Geometry: final body of the model. Coordinates: model frame, mm. Face numbers are marked on the shaded views. A direction names the side the tool comes from. Coordinates: 2 decimals unless noted, no trailing zeros. Loops run counter-clockwise (first coordinate to the right, second up) from the corner with the lowest first, then second, coordinate; pieces in that order, holes last. Notation, with made-up numbers: (-17, 47.25) - (29, 47.25) arc R26 ccw to (29, 75.25) - close; hole circle Ø8 at (27.5, -11.5). An arc over 180 degrees is marked (long way). Write each question's results on one line, items separated by ' | '. Start each with the question number.
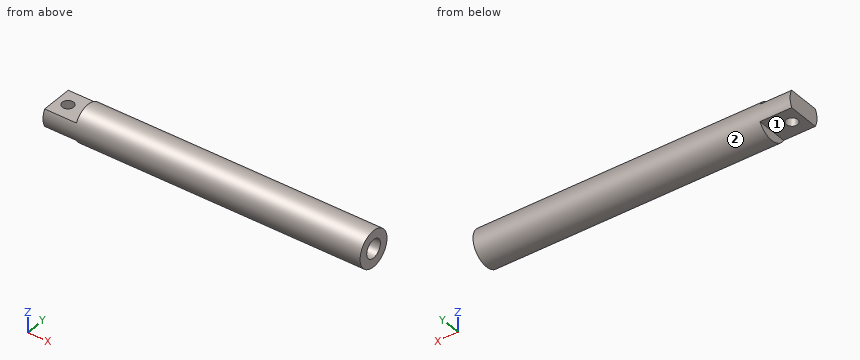
from build123d import *

# Parameters (mm, degrees)
CROQUIS1_R              = 12.5
SALIENTE_EXTRUIR1_DEPTH = 220
CROQUIS2_W              = 7.84246484
CROQUIS2_H              = 28.503577792
CROQUIS2_W_2            = 7.563798576
CROQUIS2_H_2            = 29.299767116
CORTAR_EXTRUIR1_DEPTH   = 22
CROQUIS3_R              = 3.96875
CORTAR_EXTRUIR2_DEPTH   = 22
CROQUIS4_R              = 6.35
CORTAR_EXTRUIR3_DEPTH   = 140


with BuildPart() as part:
    # Croquis1 → Saliente-Extruir1 (new body)
    with BuildSketch(Plane(origin=(0, 0, 0), x_dir=(0, 0, -1), z_dir=(1, 0, 0))):
        Circle(CROQUIS1_R)
    extrude(amount=SALIENTE_EXTRUIR1_DEPTH)

    # Croquis2 → Cortar-Extruir1 (cut)
    with BuildSketch(Plane.ZY):
        with Locations((-9.92123242, 0.389210904)):
            Rectangle(CROQUIS2_W, CROQUIS2_H)
        with Locations((9.781899288, 0.787305566)):
            Rectangle(CROQUIS2_W_2, CROQUIS2_H_2)
    extrude(amount=-CORTAR_EXTRUIR1_DEPTH, mode=Mode.SUBTRACT)

    # Croquis3 → Cortar-Extruir2 (cut)
    with BuildSketch(Plane.XY.offset(6)):
        with Locations((8, 0)):
            Circle(CROQUIS3_R)
    extrude(amount=-CORTAR_EXTRUIR2_DEPTH, mode=Mode.SUBTRACT)

    # Croquis4 → Cortar-Extruir3 (cut)
    with BuildSketch(Plane(origin=(220, 0, 0), x_dir=(0, 0, -1), z_dir=(1, 0, 0))):
        Circle(CROQUIS4_R)
    extrude(amount=-CORTAR_EXTRUIR3_DEPTH, mode=Mode.SUBTRACT)


solid = part.part
1) Access query for the marked faces 1 and 2. Directions: +Z, -Z, +X, -X, +Y, -Y. A direction counts if a zero-diameter tool reaches every point of the face in a straight line with its end or side. Return the directions, or none.
2) Section query C-C on z = -4. Output: boundary loops of the cut face in (x, y).
3) Section query D-D on x = 103. Output: boundary loops of the cut face in (y, z), and give its area (3 significant figures).
4) Pin query (flat end, axial travel): pin 1 Ø4 at (x, z) = (52, 4.5) entering from +Y; pin 2 Ø4 at (x, z) = (83.5, -3.5) entering from -Y; pin 3 Ø7 at (y, z) = (0.5, 10.5) entering from -X; pin 4 Ø14 at (y, z) = (3, 1.5) entering from +X. Return the tip coordinate at first contact, or that it passes through.
5) Section query B-B on x = 8. Output: boundary loops of the cut face in (y, z), and give its area (3 significant figures).
6) Section query A-A on y = 0. Output: boundary loops of the cut face in (x, z), and give its area (3 significant figures).
7) Material intervals for line 1 (Y direction, x = 164, z = 0); line 2 (X direction, y = -2.75, z = 8.5); line 3 (Z direction, x = 153.5, y = -3.75), sorted ascending. Write a range as [from, to].
Returned:
1) face 1: -Z, -X, +Y, -Y | face 2: +X, -X
2) outline: (0, -11.84) - (220, -11.84) - (220, -4.93) - (80, -4.93) - (80, 4.93) - (220, 4.93) - (220, 11.84) - (0, 11.84) - close; hole circle Ø7.94 at (8, 0)
3) outline: circle Ø25 at (0, 0); hole circle Ø12.7 at (0, 0) | area: 364 mm²
4) pin 1: stops at y = 12.25 | pin 2: stops at y = -12.41 | pin 3: stops at x = 22 | pin 4: stops at x = 220
5) outline: (-10.97, -6) - (-3.97, -6) - (-3.97, 6) - (-10.97, 6) arc R12.5 ccw to start; (3.97, -6) - (10.97, -6) arc R12.5 ccw to (10.97, 6) - (3.97, 6) - close | area: 193 mm²
6) outline: (0, -6) - (4.03, -6) - (4.03, 6) - (0, 6) - close; (11.97, -6) - (22, -6) - (22, -12.5) - (220, -12.5) - (220, -6.35) - (80, -6.35) - (80, 6.35) - (220, 6.35) - (220, 12.5) - (22, 12.5) - (22, 6) - (11.97, 6) - close | area: 3,340 mm²
7) line 1: y = [-12.5, -6.35], [6.35, 12.5] | line 2: x = [22, 220] | line 3: z = [-11.92, -5.12], [5.12, 11.92]
